The listing builds one solid part. Answer for the finished solid, in the listing's coordinates (mm). A direction names the side the tool comes from. Coordinates: 2 decimals unless noted, no trailing zeros. Loops run counter-clockwise (first coordinate to the right, second up) from the corner with the lowest first, then second, coordinate; pieces in that order, holes last. Notation, with made-up numbers: M -8,29.5 L 17,29.5 A32 cw 17,55.5 Z; hole C 49,61.5 d5. An arc over 180 degrees is marked long. Return JSON: item names as keys, results as strings. Group by question number.
1. Section A-A (y = 0) is taken. Write down the section's boundary in (x, z) (3 decimals).
2. Section D-D (z = 31.5) is taken. Write down the section's boundary in (x, y) (3 decimals), then the cut area to 3 significant figures.
3. The mould has two halves that part along X. Classify faces 1 (the face through (-8, -3, 40)), 2 (the face through (-14.223, -5.958, 44.145)), 3 (the face through (-10.65, 5.96, 38.33)): pulls with the +X half, pulls with the -X half, needs draft (parallel to the pull), parting line crosses it, or undercut.
4. Straight lines are drawn through the part: L1, parallel to Z at x = -0.5, y = -1; L2, parallel to Z at x = 9, y = -2; L3, parallel to Y at x = -13.5, z = 40.5. For each, find the intervals that lie inside material, in ascending order. Write a range as from..to.
5. Given P1, Ø4, axis at x = 1.875, y = 0, coming from the -Z side; P2, Ø5.5, axis at x = 1.875, y = 0, coming from the +Z side; P3, Ø4.5, axis at y = -6, z = 40.5, coming from the +X side (3 decimals), each flat-ended and moving along its own axis, determine where each tip first touches the part or whether it passes through.
6. Section B-B (z = 40) is taken. Write down the section's boundary in (x, y) (3 decimals).
7. Which of the six approach directions +Z, -Z, +X, -X, +Y, -Y give full straight-line access (tool end or side, diameter ignored) to faces 4 (the face through (-9.223, 0.042, 34.145)), 5 (the face through (6.371, 7.574, 32.535)), 6 (the face through (-10.125, 0, 20))?
8. Section C-C (y = -2.5) is taken. Write down the section's boundary in (x, z) (3 decimals), then the cut area to 3 significant figures.
```python
from build123d import *

# Parameters (mm, degrees)
SKETCH1_W               = 20.25
SKETCH1_H               = 18
BOSS_EXTRUDE1_DEPTH     = 5
SKETCH2_W               = 5
SKETCH2_H               = 18
BOSS_EXTRUDE2_DEPTH     = 25
SKETCH3_W               = 18
SKETCH3_H               = 18
BOSS_EXTRUDE3_DEPTH     = 5
CUT_EXTRUDE2_DEPTH      = 33.916798523
CUT_EXTRUDE2_DEPTH_BACK = 33.916798523
SKETCH5_R               = 1.65
FILLET1_R               = 9
FILLET7_R               = 5
CUT_EXTRUDE4_DEPTH      = 41.638843795
CUT_EXTRUDE4_DEPTH_BACK = 41.638843795
SKETCH10_R              = 1.65
SKETCH10_4_R            = 3.5
SKETCH10_4_R_2          = 1.65
BOSS_EXTRUDE7_DEPTH     = 18
FILLET13_R              = 1
FILLET16_R              = 2
SKETCH11_W              = 12
SKETCH11_H              = 6
BOSS_EXTRUDE8_DEPTH     = 10
CUT_EXTRUDE5_DEPTH      = 51.771701025
CUT_EXTRUDE5_DEPTH_BACK = 51.771701025
SKETCH12_R              = 1.75
FILLET17_R              = 3
FILLET19_R              = 3
FILLET20_R              = 2


with BuildPart() as part:
    # Sketch1 → Boss-Extrude1 (new body)
    with BuildSketch(Plane.XY):
        Rectangle(SKETCH1_W, SKETCH1_H)
    extrude(amount=BOSS_EXTRUDE1_DEPTH)

    # Sketch2 → Boss-Extrude2 (add)
    with BuildSketch(Plane.XY.offset(5)):
        with Locations((-7.625, 0)):
            Rectangle(SKETCH2_W, SKETCH2_H)
    extrude(amount=BOSS_EXTRUDE2_DEPTH)

    # Sketch3 → Boss-Extrude3 (add)
    with BuildSketch(Plane.XY.offset(30)):
        with Locations((-1.125, 0)):
            Rectangle(SKETCH3_W, SKETCH3_H)
    extrude(amount=BOSS_EXTRUDE3_DEPTH)

    # Sketch5 → Cut-Extrude2 (cut, two sides: drawn at the far end of the back side and taken through both)
    with BuildSketch(Plane(origin=(0, 0, 30), x_dir=(-1, 0, 0), z_dir=(0, 0, -1)).offset(-CUT_EXTRUDE2_DEPTH_BACK)):
        with Locations((-1.875, 0)):
            Circle(SKETCH5_R)
    extrude(amount=CUT_EXTRUDE2_DEPTH + CUT_EXTRUDE2_DEPTH_BACK, mode=Mode.SUBTRACT)

    # Fillet1
    fillet1_edges = [part.edges().sort_by_distance(p)[0] for p in [
        (-10.125, 0, 0),
    ]]
    fillet(fillet1_edges, radius=FILLET1_R)

    # Fillet7
    fillet7_edges = [part.edges().sort_by_distance(p)[0] for p in [
        (7.875, -9, 32.5),
        (7.875, 9, 32.5),
    ]]
    fillet(fillet7_edges, radius=FILLET7_R)

    # Sketch10 → Cut-Extrude4 (cut, two sides: drawn at the far end of the back side and taken through both)
    with BuildSketch(Plane.XZ.offset(9).offset(-CUT_EXTRUDE4_DEPTH_BACK)):
        with Locations((9, 2.5)):
            Circle(SKETCH10_R)
    extrude(amount=CUT_EXTRUDE4_DEPTH + CUT_EXTRUDE4_DEPTH_BACK, mode=Mode.SUBTRACT)

    # Sketch10_4 → Boss-Extrude7 (add)
    with BuildSketch(Plane.XZ.offset(9)):
        with Locations((9, 2.5)):
            Circle(SKETCH10_4_R)
        with Locations(Location((9, 2.5, 0), (0, 0, 270))):
            Circle(SKETCH10_4_R_2, mode=Mode.SUBTRACT)
    extrude(amount=-BOSS_EXTRUDE7_DEPTH)

    # Fillet13
    fillet13_edges = [part.edges().sort_by_distance(p)[0] for p in [
        (6.550510257, 0, 0),
        (6.550510257, 0, 5),
    ]]
    fillet(fillet13_edges, radius=FILLET13_R)

    # Fillet16
    fillet16_edges = [part.edges().sort_by_distance(p)[0] for p in [
        (-5.125, 0, 5),
    ]]
    fillet(fillet16_edges, radius=FILLET16_R)

    # Sketch11 → Boss-Extrude8 (add)
    with BuildSketch(Plane.XY.offset(35)):
        with Locations((-9.125, 6)):
            Rectangle(SKETCH11_W, SKETCH11_H)
        with Locations((-9.125, -6)):
            Rectangle(SKETCH11_W, SKETCH11_H)
    extrude(amount=BOSS_EXTRUDE8_DEPTH)

    # Sketch12 → Cut-Extrude5 (cut, two sides: drawn at the far end of the back side and taken through both)
    with BuildSketch(Plane(origin=(0, 9, 0), x_dir=(1, 0, 0), z_dir=(0, 1, 0)).offset(-CUT_EXTRUDE5_DEPTH_BACK)):
        with Locations(Location((-10.125, -40, 0), (0, 0, 90))):
            Circle(SKETCH12_R)
    extrude(amount=CUT_EXTRUDE5_DEPTH + CUT_EXTRUDE5_DEPTH_BACK, mode=Mode.SUBTRACT)

    # Fillet17
    fillet17_edges = [part.edges().sort_by_distance(p)[0] for p in [
        (-10.125, -6, 35),
        (-15.125, 6, 45),
        (-3.125, 6, 35),
        (-3.125, 6, 45),
        (-3.125, -6, 35),
        (-3.125, -6, 45),
        (-15.125, -6, 45),
        (-10.125, 6, 35),
    ]]
    fillet(fillet17_edges, radius=FILLET17_R)

    # Fillet19
    fillet19_edges = [part.edges().sort_by_distance(p)[0] for p in [
        (-10.125, 0, 35),
    ]]
    fillet(fillet19_edges, radius=FILLET19_R)

    # Fillet20
    fillet20_edges = [part.edges().sort_by_distance(p)[0] for p in [
        (-5.125, 0, 30),
    ]]
    fillet(fillet20_edges, radius=FILLET20_R)


solid = part.part
```
Worked out:
{
 "1": {"outline": "M -10.125,9 A9 ccw -1.125,0 L 0.225,0 L 0.225,5 L -3.125,5 A2 cw -5.125,7 L -5.125,28 A2 cw -3.125,30 L 0.225,30 L 0.225,35 L -7.125,35 A3 ccw -10.125,32 Z; M 3.525,0 L 6.172,0 A1 cw 6.8,-0.222 A3.5 ccw long 6.8,5.222 A1 cw 6.172,5 L 3.525,5 Z; M 3.525,30 L 7.875,30 L 7.875,35 L 3.525,35 Z; hole C 9,2.5 d3.3"},
 "2": {"outline": "M -10.125,-9 L 2.875,-9 A5 ccw 7.875,-4 L 7.875,4 A5 ccw 2.875,9 L -10.125,9 Z; hole C 1.875,0 d3.3", "area": "305 mm^2"},
 "3": {"face 1": "needs draft", "face 2": "pulls with the -X half", "face 3": "undercut"},
 "4": {"L1": "0..5, 30..35", "L2": "-1..0.85, 4.15..6", "L3": "-9..-3, 3..9"},
 "5": {"P1": "z = 0", "P2": "z = 35", "P3": "x = -3.125"},
 "6": {"outline": "M -15.125,-9 L -11.875,-9 L -11.875,-3 L -15.125,-3 Z; M -15.125,3 L -11.875,3 L -11.875,9 L -15.125,9 Z; M -8.375,-9 L -3.125,-9 L -3.125,-3 L -8.375,-3 Z; M -8.375,3 L -3.125,3 L -3.125,9 L -8.375,9 Z"},
 "7": {"face 4": "+Z, -X", "face 5": "+Z, +X, +Y", "face 6": "-Z, -X, +Y, -Y"},
 "8": {"outline": "M -10.125,9 A9 ccw -1.125,0 L 6.172,0 A1 cw 6.8,-0.222 A3.5 ccw long 6.8,5.222 A1 cw 6.172,5 L -3.125,5 A2 cw -5.125,7 L -5.125,28 A2 cw -3.125,30 L 7.875,30 L 7.875,35 L -7.125,35 A3 ccw -10.125,32 Z; hole C 9,2.5 d3.3", "area": "307 mm^2"}
}
